Can you work these out from the drawing? Everything is in mm from the part's minimum corner. A direction names the side the tool comes from. Give positions to 0.01 mm unless a question says otherwise; leave off trailing zeros. Order: outer loops, then holes, each group sorted by start corner. A loop starts at its lowest first (then second) coordinate and runs counter-clockwise, first axis right, second up. Notation, with made-up numbers: M 54.5,44 L 83.5,44 A15 ccw 83.5,71 Z; hole C 1,26 d1. An arc over 180 degrees is marked long. Use a Markdown table: item, result. Add a question column.
Item 1: For the marked faces 1 and 2, which set-ups out of +Z, -Z, +X, -X, +Y, -Y let a thin tool reach every point of the face, with its end or its side?
Item 2: I'm going to push flat-ended pins straight in: pin 1 Ø1 at (y, z) = (17, 4.5) entering from -X; pin 2 Ø3 at (y, z) = (21.5, 10.5) entering from +X; pin 3 Ø2 at (x, z) = (60, 11.5) entering from -Y. Where does each tip first touch, or does it pass through?
Item 3: Suppose I cut it at C-C on x = 51.5. Write out the boundary of the cut face in (y, z), plus the area to 3 significant figures.
Item 4: Suppose I cut it at B-B on y = 7. Write out the boundary of the cut face in (x, z), plus the area to 3 significant figures.
Item 5: If I drill on L1, parallel to X at y = 5, z = 14.25; L2, parallel to Y at x = 14, z = 11.75; L3, parallel to Y at x = 93, z = 9.5, over which ranges is the centre line in solid material (lowest first)? Write a range as from..to.
Item 6: Suppose I cut it at A-A on z = 18.75. Write out the boundary of the cut face in (x, y).
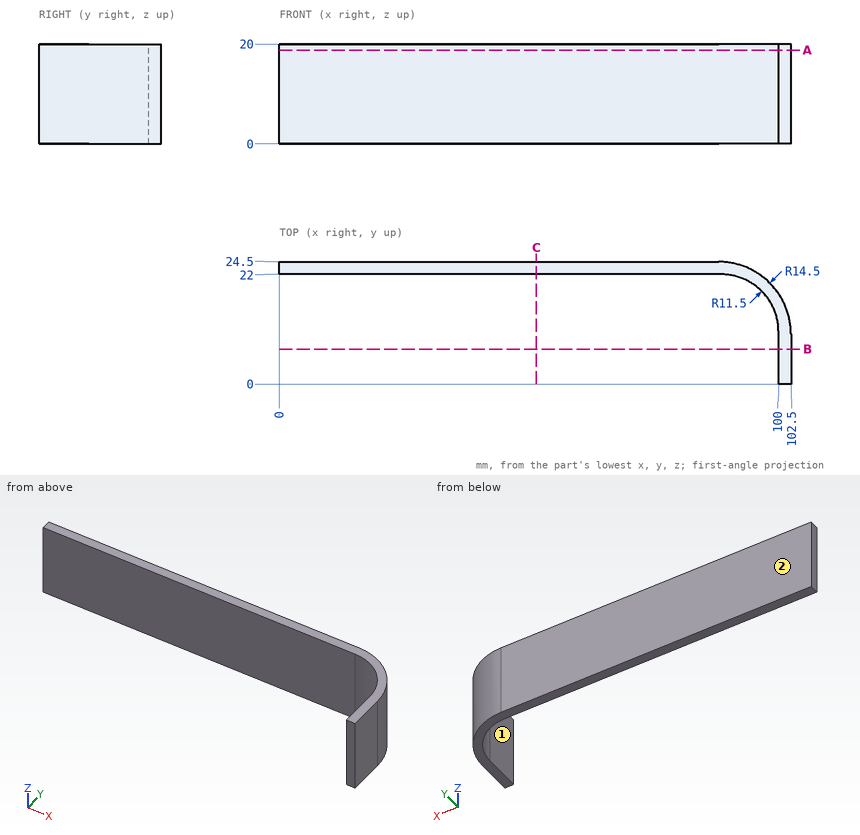
Findings below:
| question | item | result |
|---|---|---|
| 1 | face 1 | +Z, -Z, -X, -Y |
| 1 | face 2 | +Z, -Z, +X, -X, +Y |
| 2 | pin 1 | stops at x = 97.62 |
| 2 | pin 2 | stops at x = 98.5 |
| 2 | pin 3 | stops at y = 22 |
| 3 | outline | M 22,0 L 24.5,0 L 24.5,20 L 22,20 Z |
| 3 | area | 50.0 mm^2 |
| 4 | outline | M 100,0 L 102.5,0 L 102.5,20 L 100,20 Z |
| 4 | area | 50.0 mm^2 |
| 5 | L1 | x = 100..102.5 |
| 5 | L2 | y = 22..24.5 |
| 5 | L3 | y = 21.08..23.61 |
| 6 | outline | M 0,22 L 88.5,22 A11.5 cw 100,10.5 L 100,0 L 102.5,0 L 102.5,10 A14.5 ccw 88,24.5 L 0,24.5 Z |
